For this review, take the finished solid that the model builds, in its own axes (mm). Face numbers are marked on the shaded views. Round coordinates to 2 decimals unless told otherwise and drop trailing zeros. Order: outer loops, then holes, each group sorted by start corner. A loop starts at its lowest first (then second) coordinate and runs counter-clockwise, first axis right, second up. Notation, with made-up numbers: M 23.25,-11 L 67.25,-11 A22 ccw 67.25,5 Z; hole C -26,43 d8. An arc over 180 degrees is marked long. Answer as a JSON object with one key per item and string values.
from build123d import *

# Parameters (mm, degrees)
SKETCH1_R           = 25.146
BOSS_EXTRUDE1_DEPTH = 14.224
CUT_EXTRUDE1_REACH  = 16.224
SKETCH2_R           = 1.397
CUT_EXTRUDE2_REACH  = 16.224
SKETCH3_R           = 16.383


with BuildPart() as part:
    # Sketch1 → Boss-Extrude1 (new body)
    with BuildSketch(Plane(origin=(0, 0, 0), x_dir=(1, 0, 0), z_dir=(0, 1, 0))):
        Circle(SKETCH1_R)
    extrude(amount=BOSS_EXTRUDE1_DEPTH)

    # Sketch2 → Cut-Extrude1 (cut, up to next)
    with BuildSketch(Plane(origin=(0, 14.224, 0), x_dir=(1, 0, 0), z_dir=(0, 1, 0)), mode=Mode.PRIVATE) as cut_extrude1_sk1:
        with Locations((13.97, 13.97)):
            Circle(SKETCH2_R)
    cut_extrude1_tool1 = extrude(cut_extrude1_sk1.sketch, amount=-CUT_EXTRUDE1_REACH, mode=Mode.PRIVATE) & part.part
    add(cut_extrude1_tool1.solids().sort_by_distance((13.97, 14.224, -13.97))[0], mode=Mode.SUBTRACT)
    # Sketch2 → Cut-Extrude1 (cut, up to next)
    with BuildSketch(Plane(origin=(0, 14.224, 0), x_dir=(1, 0, 0), z_dir=(0, 1, 0)), mode=Mode.PRIVATE) as cut_extrude1_sk2:
        with Locations((13.97, -13.97)):
            Circle(SKETCH2_R)
    cut_extrude1_tool2 = extrude(cut_extrude1_sk2.sketch, amount=-CUT_EXTRUDE1_REACH, mode=Mode.PRIVATE) & part.part
    add(cut_extrude1_tool2.solids().sort_by_distance((13.97, 14.224, 13.97))[0], mode=Mode.SUBTRACT)
    # Sketch2 → Cut-Extrude1 (cut, up to next)
    with BuildSketch(Plane(origin=(0, 14.224, 0), x_dir=(1, 0, 0), z_dir=(0, 1, 0)), mode=Mode.PRIVATE) as cut_extrude1_sk3:
        with Locations((-13.97, -13.97)):
            Circle(SKETCH2_R)
    cut_extrude1_tool3 = extrude(cut_extrude1_sk3.sketch, amount=-CUT_EXTRUDE1_REACH, mode=Mode.PRIVATE) & part.part
    add(cut_extrude1_tool3.solids().sort_by_distance((-13.97, 14.224, 13.97))[0], mode=Mode.SUBTRACT)
    # Sketch2 → Cut-Extrude1 (cut, up to next)
    with BuildSketch(Plane(origin=(0, 14.224, 0), x_dir=(1, 0, 0), z_dir=(0, 1, 0)), mode=Mode.PRIVATE) as cut_extrude1_sk4:
        with Locations((-13.97, 13.97)):
            Circle(SKETCH2_R)
    cut_extrude1_tool4 = extrude(cut_extrude1_sk4.sketch, amount=-CUT_EXTRUDE1_REACH, mode=Mode.PRIVATE) & part.part
    add(cut_extrude1_tool4.solids().sort_by_distance((-13.97, 14.224, -13.97))[0], mode=Mode.SUBTRACT)

    # Sketch3 → Cut-Extrude2 (cut, up to next)
    with BuildSketch(Plane(origin=(0, 14.224, 0), x_dir=(1, 0, 0), z_dir=(0, 1, 0)), mode=Mode.PRIVATE) as cut_extrude2_sk1:
        Circle(SKETCH3_R)
    cut_extrude2_tool1 = extrude(cut_extrude2_sk1.sketch, amount=-CUT_EXTRUDE2_REACH, mode=Mode.PRIVATE) & part.part
    add(cut_extrude2_tool1.solids().sort_by_distance((0, 14.224, 0))[0], mode=Mode.SUBTRACT)


solid = part.part
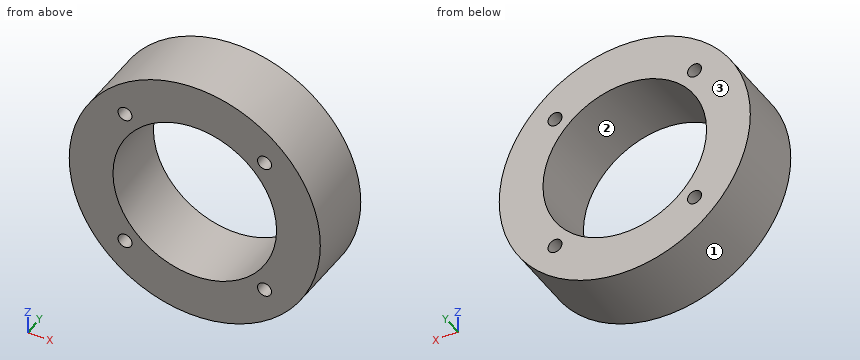
1) Insertion check: P1, Ø8, axis at x = 4.5, y = 7, coming from the +Z side; P2, Ø2, axis at y = 3.5, z = 5.5, coming from the +X side; P3, Ø8, axis at x = 8.5, y = 2.5, coming from the -Z side. Each pin has a flat end and moves straight along its axis. Give the tip position at first contact, or say it passes through.
Geometry check:
{"P1": "stops at z = 25.14", "P2": "stops at x = 24.74", "P3": "stops at z = -24.74"}
2) Add section B-B on z = 0. State the section outline as (x, y) points, and give its area (3 significant figures).
Geometry check:
{"outline": "M -25.15,0 L -16.38,0 L -16.38,14.22 L -25.15,14.22 Z; M 16.38,0 L 25.15,0 L 25.15,14.22 L 16.38,14.22 Z", "area": "249 mm²"}
3) Add section C-C on x = 14. State the section outline as (y, z) points.
Geometry check:
{"outline": "M 0,-20.89 L 14.22,-20.89 L 14.22,-15.37 L 0,-15.37 Z; M 0,-12.57 L 14.22,-12.57 L 14.22,-8.51 L 0,-8.51 Z; M 0,8.51 L 14.22,8.51 L 14.22,12.57 L 0,12.57 Z; M 0,15.37 L 14.22,15.37 L 14.22,20.89 L 0,20.89 Z"}
4) Add section A-A on x = 0. State the section outline as (y, z) points.
Geometry check:
{"outline": "M 0,-25.15 L 14.22,-25.15 L 14.22,-16.38 L 0,-16.38 Z; M 0,16.38 L 14.22,16.38 L 14.22,25.15 L 0,25.15 Z"}
5) For L1, parallel to Z at x = 13.97, y = 6.5; L2, parallel to X at y = 8.75, z = 0, list the stretches that pass through material, from the lowest coordinate up.
Geometry check:
{"L1": "z = -20.91 to -15.37, -12.57 to -8.56, 8.56 to 12.57, 15.37 to 20.91", "L2": "x = -25.15 to -16.38, 16.38 to 25.15"}
6) Mouldability with a two-part tool opening along Z and no side actions: class the marked faces 1, 2 and 3 as +Z half, -Z half, draft (parallel to the pull), parting line (faces both ways), or undercut.
Geometry check:
{"face 1": "parting line", "face 2": "undercut", "face 3": "draft"}
7) Add section D-D on y = 6. State the section outline as (x, z) points.
Geometry check:
{"outline": "C 0,0 d50.29; hole C 0,0 d32.77; hole C -13.97,-13.97 d2.79; hole C -13.97,13.97 d2.79; hole C 13.97,-13.97 d2.79; hole C 13.97,13.97 d2.79"}
